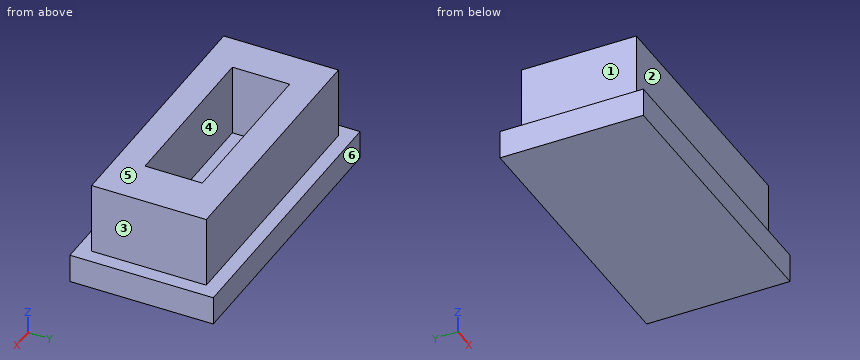
from build123d import *

# Parameters (mm, degrees)
F0_W     = 100
F0_H     = 50
F1_DEPTH = 10
F2_W     = 90
F2_H     = 40
F3_DEPTH = 5
F4_DEPTH = 25
F5_W     = 59.516436
F5_H     = 20
F6_DEPTH = 25


with BuildPart() as f1:
    # F0 (on Top) → F1 (new body)
    with BuildSketch(Plane.XY):
        with Locations((-0.379814, -32.520819)):
            Rectangle(F0_W, F0_H)
    extrude(amount=F1_DEPTH)

    # F2 (on face) → F3 (join)
    with BuildSketch(Plane.XY.offset(10)):
        with Locations((-0.379814, -32.520819)):
            Rectangle(F2_W, F2_H)
    extrude(amount=F3_DEPTH)

    # F2 (on face) → F4 (join)
    with BuildSketch(Plane.XY.offset(10)):
        with Locations((-0.379814, -32.520819)):
            Rectangle(F2_W, F2_H)
    extrude(amount=F4_DEPTH)

    # F5 (on face) → F6 (cut)
    with BuildSketch(Plane.XY.offset(35)):
        with Locations((-1.975571, -32.520819)):
            Rectangle(F5_W, F5_H)
    extrude(amount=-F6_DEPTH, mode=Mode.SUBTRACT)


solid = f1.part
Model file for the job. Use its own axes, mm. Face numbers are marked on the shaded views. A direction names the side the tool comes from. Give positions to 0.01 mm unless a question says otherwise; leave off trailing zeros. Order: outer loops, then holes, each group sorted by start corner. A loop starts at its lowest first (then second) coordinate and runs counter-clockwise, first axis right, second up. Notation, with made-up numbers: (-19, -17.5) - (10, -17.5) arc R25 cw to (10, 5.5) - close; hole circle Ø8 at (16.25, 85). An arc over 180 degrees is marked (long way). One line per item, written item: value.
Item 1: Slice it at D-D (x = -35.5). List the corners of the cut face in (y, z).
Response values:
outline: (-57.52, 0) - (-7.52, 0) - (-7.52, 10) - (-12.52, 10) - (-12.52, 35) - (-52.52, 35) - (-52.52, 10) - (-57.52, 10) - close
Item 2: Slice it at B-B (x = -4). List the corners of the cut face in (y, z), then the cut area to 3 significant figures.
Response values:
outline: (-57.52, 0) - (-7.52, 0) - (-7.52, 10) - (-12.52, 10) - (-12.52, 35) - (-22.52, 35) - (-22.52, 10) - (-42.52, 10) - (-42.52, 35) - (-52.52, 35) - (-52.52, 10) - (-57.52, 10) - close
area: 1,000 mm2
Item 3: Slice it at A-A (z = 21). List the corners of the cut face in (x, y), then the cut area to 3 significant figures.
Response values:
outline: (-45.38, -52.52) - (44.62, -52.52) - (44.62, -12.52) - (-45.38, -12.52) - close; hole (-31.73, -42.52) - (27.78, -42.52) - (27.78, -22.52) - (-31.73, -22.52) - close
area: 2,410 mm2
Item 4: Slice it at C-C (y = -36.5). List the corners of the cut face in (x, z), then the cut area to 3 significant figures.
Response values:
outline: (-50.38, 0) - (49.62, 0) - (49.62, 10) - (44.62, 10) - (44.62, 35) - (27.78, 35) - (27.78, 10) - (-31.73, 10) - (-31.73, 35) - (-45.38, 35) - (-45.38, 10) - (-50.38, 10) - close
area: 1,760 mm2
Item 5: Pin check, flat tips, straight feed: pin 1 Ø8 at (y, z) = (-38.5, 23.5) entering from +X; pin 2 Ø7.5 at (x, z) = (-8, 22) entering from +Y; pin 3 Ø12.5 at (y, z) = (-32, 25.5) entering from -X. Stop position of each tip, or through.
Response values:
pin 1: x = 44.62
pin 2: y = -12.52
pin 3: x = -45.38
Item 6: Wall check: line 1 (Y direction, x = -8.5, z = 18); line 2 (X direction, y = -34, z = 11); line 3 (X direction, y = -13, z = 34). Give the ranges that are in metal, low to high.
Response values:
line 1: -52.52 to -42.52, -22.52 to -12.52
line 2: -45.38 to -31.73, 27.78 to 44.62
line 3: -45.38 to 44.62
Item 7: Tool access for the marked faces 1, 2 and 3: list every direction of +Z, -Z, +X, -X, +Y, -Y with a clear straight run to the whole face (end or side of a thin tool).
Response values:
face 1: +Z, -X, +Y, -Y
face 2: +Z, +X, -X, -Y
face 3: +Z, +X, +Y, -Y
Item 8: Two-plate mould, pull along Y, no slides. Class the marked faces 4, 5 and 6: released by +Y, released by -Y, zero draft, split by the parting line, or undercut.
Response values:
face 4: undercut
face 5: zero draft
face 6: released by +Y
